Autodesk Inventor part; units mm, degrees
ref_plane "YZ Plane" through (0, 0, 0) normal (1, 0, 0) x (0, 1, 0)
ref_plane "XZ Plane" through (0, 0, 0) normal (0, 1, 0) x (-1, 0, 0)
ref_plane "XY Plane" through (0, 0, 0) normal (0, 0, 1) x (1, 0, 0)
sketch "Эскиз1" plane through (0, 0, 0) normal (0, 0, 1) x (1, 0, 0)
  line L0 (-70, 0) -> (70, 0)
  line L1 (70, 0) -> (70, 10)
  line L2 (70, 10) -> (-70, 10)
  line L3 (-70, 10) -> (-70, 0)
  line L4 (-70, 0) -> (-84, 0)
  line L5 (-84, 0) -> (-84, 60)
  line L6 (-84, 60) -> (-70, 60)
  line L7 (-70, 60) -> (-70, 0)
  line L8 (-70, 50) -> (-70, 60)
  line L9 (-70, 40) -> (70, 40)
  line L10 (70, 40) -> (70, 50)
  line L11 (70, 50) -> (-70, 50)
  line L12 (-70, 50) -> (-70, 40)
  line L13 (70, 0) -> (84, 0)
  line L14 (84, 0) -> (84, 60)
  line L15 (84, 60) -> (70, 60)
  line L16 (70, 60) -> (70, 0)
  line L17 (-55, 40) -> (-25, 10)
  line L18 (-40.8579, 40) -> (-10.8579, 10)
  line L19 (55, 40) -> (25, 10)
  line L20 (10.8579, 10) -> (40.8579, 40)
  point P0 (0, 0)
  dimension "d0" = 140
  dimension "d1" = 10
  dimension "d2" = 60
  dimension "d4" = 10
  dimension "d5" = 10
  dimension "d6" = 60
  dimension "d7" = 14
  dimension "d8" = 14
  dimension "d9" = 0
  dimension "d24" = 45
  dimension "d25" = 45
  dimension "d26" = 10
  dimension "d27" = 0
  dimension "d28" = 15
  dimension "d29" = 70
  dimension "d30" = 45
  dimension "d31" = 45
  dimension "d32" = 15
  dimension "d33" = 10
extrude "Выдавливание1" add sketch "Эскиз1" against normal blind 3 contours L3 L2 L1 L0 | L4 L5 L6 L7 L3 | L1 L16 L10 L15 L14 L13 | L17 L9 L18 L2 | L7 L11 L10 L9 | L2 L20 L9 L19
sketch "Эскиз2" plane through (0, 0, -3) normal (0, 0, -1) x (-1, 0, 0)
  line L0 (-70, 60) -> (-84, 60)
  line L1 (-70, 60) -> (-71, 60)
  line L2 (-71, 60) -> (-71, 0)
  line L3 (-71, 0) -> (-70, 0)
  line L4 (-70, 0) -> (-70, 60)
  line L5 (70, 60) -> (71, 60)
  line L6 (71, 60) -> (71, 0)
  line L7 (71, 0) -> (70, 0)
  line L8 (70, 0) -> (70, 60)
  line L9 (-84, 0) -> (84, 0)
  point P0 (0, 0)
  dimension "d12" = 1
  dimension "d13" = 1
  dimension "d34" = 0
extrude "Выдавливание2" add sketch "Эскиз2" along normal blind 9
fillet "Сопряжение1" radius 13 2 edges at (71, 30, -3) (-71, 30, -3)
chamfer "Фаска2" distance 4 angle 45 14 edges at (-70, 50, -1.5) (-70, 10, -1.5) (-70, 40, -1.5) (70, 10, -1.5) (70, 40, -1.5) (70, 50, -1.5) (25, 10, -1.5) (-10.8579, 10, -1.5) (40.8579, 40, -1.5) (-25, 10, -1.5) (10.8579, 10, -1.5) (-40.8579, 40, -1.5) (-55, 40, -1.5) (55, 40, -1.5)
chamfer "Фаска3" distance 4 angle 45 8 edges at (-70, 52, -3) (-70, 38, -3) (-70, 5, -3) (-70, 12, -3) (70, 52, -3) (70, 38, -3) (70, 5, -3) (70, 12, -3)
fillet "Сопряжение2" radius 15 2 edges at (-84, 30, 0) (84, 30, 0)
properties part number "zenter"
The listing builds one solid part. Answer for the finished solid, in the listing's coordinates (mm). A direction names the side the tool comes from. Give positions to 0.01 mm unless a question says otherwise; leave off trailing zeros. Write each loop counter-clockwise with the first axis right and the second up, starting at its lowest first coordinate (ties: lowest second). Pieces come first, ordered by that corner, then holes. Notation, with made-up numbers: (-14, 16.5) - (1, 16.5) arc R34 cw to (1, 47.5) - close; hole circle Ø7 at (14, 58). An arc over 180 degrees is marked (long way). Use one line per item in the form item = value. Start each with the question number.
1) Flat-ended cylindrical pins translate along their axes: pin 1 Ø4 at (x, y) = (57.5, 44.5) entering from -Z; pin 2 Ø0.9 at (x, z) = (-52.5, -1.5) entering from +Y. Find the tip coordinate at first contact, or state that the pin passes through.
2) Find section A-A on x = 47.5. Determine the outline of the cut face in (y, z), plus the area to 3 significant figures.
3) Consider line 1 along X through (y, z) = (22, -1.25); line 2 along X through (y, z) = (26.5, -11.5); line 3 along X through (y, z) = (27, -5.25). Determine where each line is inside the solid, lowest interval first. Write a range as from..to.
4) The mould has two halves that part along X. Classify faces 1 (the face through (0, 0, -2)), 2 (the face through (75.629, 30.42, -5.556)), 3 (the face through (28.406, 11.434, -1.479)): pulls with the +X half, pulls with the -X half, needs draft (parallel to the pull), parting line crosses it, or undercut.
5) Find section D-D on y = 30.5. Determine the outline of the cut face in (x, z), plus the area to 3 significant figures.
6) Find section B-B on z = -5.25. Determine the outline of the cut face in (x, y), plus the area to 3 significant figures.
7) Find section C-C on y = 7. Determine the outline of the cut face in (x, z), plus the area to 3 significant figures.
8) A tool of negligible diameter and unlimited length cuts with its end or side. For faces 4 (the face through (-1, 40, -1)), 5 (the face through (68, 52, -3)), 6 (the face through (70, 30, -7)), 7 (the face through (-1, 9, -3)), from which of +Z, -Z, +X, -X, +Y, -Y can it reach the whole face along a straight path? Write none if from no direction.
Geometry results:
q1.pin_1 = -3
q1.pin_2 = 50
q2.outline = (0, -3) - (10, -3) - (10, 0) - (0, 0) - close; (32.5, -3) - (50, -3) - (50, 0) - (32.5, 0) - close
q2.area = 82.5 mm2
q3.line_1 = -80.99..-70, -37..-22.86, 22.86..37, 70..80.99
q3.line_2 = -71.17..-70, 70..71.17
q3.line_3 = -76.06..-70, 70..76.06
q4.face_1 = needs draft
q4.face_2 = pulls with the +X half
q4.face_3 = undercut
q5.outline = (-84, -3) - (-83.37, -3) arc R13 cw to (-71, -12) - (-70, -12) - (-70, 0) - (-75, 0) arc R15 ccw to start; (-45.5, -3) - (-31.36, -3) - (-31.36, 0) - (-45.5, 0) - close; (31.36, -3) - (45.5, -3) - (45.5, 0) - (31.36, 0) - close; (70, -12) - (71, -12) arc R13 cw to (83.37, -3) - (84, -3) arc R15 ccw to (75, 0) - (70, 0) - close
q5.area = 229 mm2
q6.outline = (-76.06, 0) - (-68.25, 0) - (-68.25, 12.25) - (-70, 14) - (-70, 36) - (-68.25, 37.75) - (-68.25, 52.25) - (-70, 54) - (-70, 60) - (-76.06, 60) - close; (68.25, 0) - (76.06, 0) - (76.06, 60) - (70, 60) - (70, 54) - (68.25, 52.25) - (68.25, 37.75) - (70, 36) - (70, 14) - (68.25, 12.25) - close
q6.area = 830 mm2
q7.outline = (-84, -3) - (-83.37, -3) arc R13 cw to (-71, -12) - (-70, -12) - (-70, -7) - (-66, -3) - (66, -3) - (70, -7) - (70, -12) - (71, -12) arc R13 cw to (83.37, -3) - (84, -3) arc R15 ccw to (75, 0) - (-75, 0) arc R15 ccw to start
q7.area = 580 mm2
q8.face_4 = +Z, -Z
q8.face_5 = +Z, -Z, +Y
q8.face_6 = -Z
q8.face_7 = -Z, +Y, -Y
